The model under review builds one solid part; all positions refer to its coordinate system, in mm. Round coordinates to 2 decimals unless told otherwise and drop trailing zeros. Loops run counter-clockwise (first coordinate to the right, second up) from the corner with the lowest first, then second, coordinate; pieces in that order, holes last. Notation, with made-up numbers: M 84,-20 L 132,-20 A32 cw 132,10 Z; hole C 7,-3.75 d2. An arc over 180 degrees is marked long. Use a Markdown table: item, result. Add a question column.
```python
from build123d import *

# Parameters (mm, degrees)
BOSS_EXTRUDE1_DEPTH = 3.175


with BuildPart() as part:
    # Sketch1 → Boss-Extrude1 (new body)
    with BuildSketch(Plane.XY):
        with BuildLine():
            Line((-152.4, 22.70125), (-152.4, 40.64))
            Line((-152.4, 40.64), (-156.516961876, 40.022455719))
            ThreePointArc((-156.516961876, 40.022455719), (-160.386650336, 37.886442621), (-161.925, 33.742709878))
            Line((-161.925, 33.742709878), (-161.925, 6.35))
            ThreePointArc((-161.925, 6.35), (-160.065128061, 1.859871939), (-155.575, 0))
            Line((-155.575, 0), (-152.4, 0))
            Line((-152.4, 0), (-152.4, 17.93875))
            ThreePointArc((-152.4, 17.93875), (-154.78125, 20.32), (-152.4, 22.70125))
        make_face()
        with BuildLine():
            Line((-123.825, 0), (-114.3, 0))
            Line((-114.3, 0), (-114.3, 20.79625))
            ThreePointArc((-114.3, 20.79625), (-116.68125, 23.1775), (-114.3, 25.55875))
            Line((-114.3, 25.55875), (-114.3, 46.355))
            Line((-114.3, 46.355), (-152.4, 40.64))
            Line((-152.4, 40.64), (-152.4, 22.70125))
            ThreePointArc((-152.4, 22.70125), (-150.716201977, 22.003798023), (-150.01875, 20.32))
            ThreePointArc((-150.01875, 20.32), (-150.716201977, 18.636201977), (-152.4, 17.93875))
            Line((-152.4, 17.93875), (-152.4, 0))
            Line((-152.4, 0), (-136.525, 0))
            Line((-136.525, 0), (-136.525, 3.915859715))
            Line((-136.525, 3.915859715), (-123.825, 3.915859715))
            Line((-123.825, 3.915859715), (-123.825, 0))
        make_face()
        with BuildLine():
            Line((-114.3, 20.79625), (-114.3, 0))
            Line((-114.3, 0), (-111.125, 0))
            ThreePointArc((-111.125, 0), (-106.634871939, 1.859871939), (-104.775, 6.35))
            Line((-104.775, 6.35), (-104.775, 40.410209878))
            ThreePointArc((-104.775, 40.410209878), (-106.981267257, 45.221860214), (-112.066961876, 46.689955719))
            Line((-112.066961876, 46.689955719), (-114.3, 46.355))
            Line((-114.3, 46.355), (-114.3, 25.55875))
            ThreePointArc((-114.3, 25.55875), (-112.616201977, 24.861298023), (-111.91875, 23.1775))
            ThreePointArc((-111.91875, 23.1775), (-112.616201977, 21.493701977), (-114.3, 20.79625))
        make_face()
    extrude(amount=BOSS_EXTRUDE1_DEPTH)


solid = part.part
```
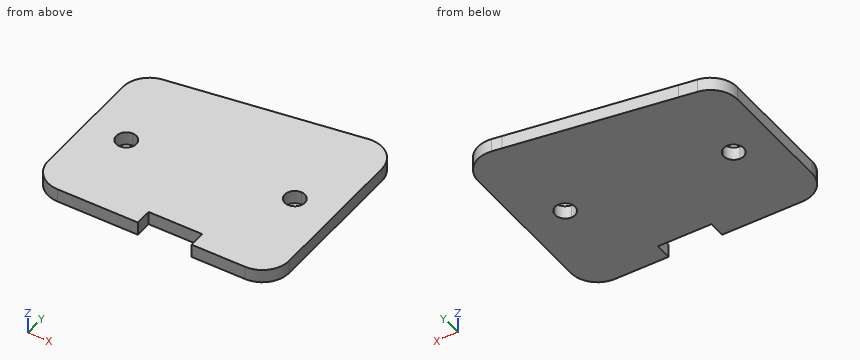
(1) Consider section B-B, the plane x = -132. Give the boundary of the cut face in (y, z) (3 decimals).
(2) Consider section C-C, the plane x = -144. Give the boundary of the cut face in (y, z) (3 decimals), then the cut area to 3 significant figures.
(3) To check wall thickness, follow probe 1 along Y at (x, z) = (-152.5, 2.4) (3 decimals); probe 2 along Y at (x, z) = (-154, 1.75); probe 3 along X at (y, z) = (21, 1.2) (3 decimals). State the ranges of each line that lie inside material, in increasing order.
(4) Insertion check: pin 1 Ø10 at (x, y) = (-147.5, 41) entering from -Z; pin 2 Ø1.6 at (y, z) = (2.5, 1) entering from -X; pin 3 Ø1.6 at (x, z) = (-133, 2) entering from -Y. Each pin has a flat end and moves straight along its axis. Give the tip position at first contact, or say it passes through.
(5) Consider section A-A, the plane z = 2.1. Give the number of separate pieces and of enclosed holes in the cut face, then the cut area to 3 significant figures.
Found:
| question | item | result |
|---|---|---|
| 1 | outline | M 3.916,0 L 43.7,0 L 43.7,3.175 L 3.916,3.175 Z |
| 2 | outline | M 0,0 L 41.9,0 L 41.9,3.175 L 0,3.175 Z |
| 2 | area | 133 mm^2 |
| 3 | probe 1 | y = 0 to 17.941, 22.699 to 40.625 |
| 3 | probe 2 | y = 0 to 18.56, 22.08 to 40.4 |
| 3 | probe 3 | x = -161.925 to -154.682, -150.118 to -115.264, -113.336 to -104.775 |
| 4 | pin 1 | stops at z = 0 |
| 4 | pin 2 | stops at x = -161.14 |
| 4 | pin 3 | stops at y = 3.92 |
| 5 | separate pieces | 1 |
| 5 | enclosed holes | 2 |
| 5 | area | 2,370 mm^2 |
